Read the model definition and answer for the solid it produces. Units are mm, in the model's axes. Face numbers are marked on the shaded views. A direction names the side the tool comes from. Give positions to 0.01 mm unless a question says otherwise; leave off trailing zeros. Order: outer loops, then holes, each group sorted by start corner. A loop starts at its lowest first (then second) coordinate and runs counter-clockwise, first axis right, second up.
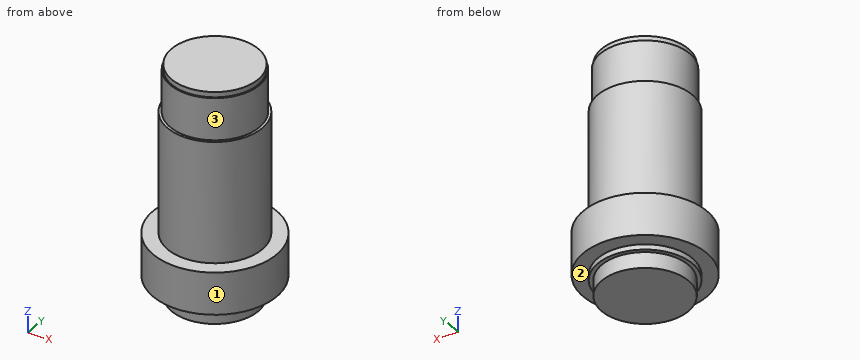
Autodesk Inventor part; units mm, degrees
ref_plane "作業平面1" through (0, 0, 4) normal (0, 0, -1) x (-1, 0, 0)
ref_plane "YZ Plane" through (0, 0, 0) normal (1, 0, 0) x (0, 1, 0)
ref_plane "XZ Plane" through (0, 0, 0) normal (0, 1, 0) x (-1, 0, 0)
sketch "スケッチ1" plane through (0, 0, 0) normal (0, 0, 1) x (1, 0, 0)
  circle A0 centre (0, 0) radius 8.25
  dimension "d0" = 16.5
extrude "押し出し1" add sketch "スケッチ1" along normal blind 3
sketch "スケッチ2" plane through (0, 0, 3) normal (0, 0, 1) x (1, 0, 0)
  circle A0 centre (0, 0) radius 9
  dimension "d3" = 18
extrude "押し出し2" add sketch "スケッチ2" along normal blind 32
sketch "スケッチ3" plane through (0, 0, 35) normal (0, 0, 1) x (1, 0, 0)
  circle A0 centre (0, 0) radius 8.5
  dimension "d6" = 17
extrude "押し出し3" add sketch "スケッチ3" along normal blind 8
sketch "スケッチ4" plane through (0, 0, 43) normal (0, 0, 1) x (1, 0, 0)
  circle A0 centre (0, 0) radius 8.25
  dimension "d9" = 16.5
extrude "押し出し4" add sketch "スケッチ4" along normal blind 1
ref_plane "作業平面1" through (0, 0, 4) normal (0, 0, -1) x (-1, 0, 0)
sketch "スケッチ6" plane through (0, 0, 4) normal (0, 0, -1) x (-1, 0, 0)
  circle A0 centre (0, 0) radius 11.75
  circle A1 centre (0, 0) radius 9
  dimension "d16" = 23.5
extrude "押し出し6" add sketch "スケッチ6" against normal blind 8
properties part number "E18_D80NK" material "ABS プラスチック"
1) Given pin 1 (8 mm diameter, centred on x = -9, z = 25.5, fed in from -Y); pin 2 (5 mm diameter, centred on x = 6.5, z = 18, fed in from -Y); pin 3 (1.5 mm diameter, centred on x = -6.5, y = 7.5, fed in from +Z); pin 4 (12 mm diameter, centred on x = -2.5, y = -8.5, fed in from -Z), each flat-ended and moving along its own axis, determine where each tip first touches the part or whether it passes through.
Final values:
pin 1: stops at y = -7.48
pin 2: stops at y = -8.06
pin 3: stops at z = 12
pin 4: stops at z = 0
2) The part is cut by section C-C on z = 32. Determine the outline of the cut face in (x, y).
Final values:
outline: circle Ø18 at (0, 0)
3) The part is cut by section D-D on z = 6. Determine the outline of the cut face in (x, y), and give its area (3 significant figures).
Final values:
outline: circle Ø23.5 at (0, 0)
area: 434 mm2
4) A tool of negligible diameter and unlimited length cuts with its end or side. For the marked faces 1, 2 and 3, from which of +Z, -Z, +X, -X, +Y, -Y can it reach the whole face along a straight path? Write none if from no direction.
Final values:
face 1: +Z, -Z
face 2: -Z
face 3: +Z
5) The part is cut by section A-A on y = 0. Determine the outline of the cut face in (x, z), and give its area (3 significant figures).
Final values:
outline: (-11.75, 4) - (-9, 4) - (-9, 3) - (-8.25, 3) - (-8.25, 0) - (8.25, 0) - (8.25, 3) - (9, 3) - (9, 4) - (11.75, 4) - (11.75, 12) - (9, 12) - (9, 35) - (8.5, 35) - (8.5, 43) - (8.25, 43) - (8.25, 44) - (-8.25, 44) - (-8.25, 43) - (-8.5, 43) - (-8.5, 35) - (-9, 35) - (-9, 12) - (-11.75, 12) - close
area: 822 mm2
6) Consider L1, parallel to Y at x = -0.25, z = 25; L2, parallel to Y at x = 0.5, z = 10; L3, parallel to Z at x = 9.25, y = -4.5. Determine where each line is inside the solid, lowest interval first.
Final values:
L1: y = -9 to 9
L2: y = -11.74 to 11.74
L3: z = 4 to 12
